Autodesk Inventor part; units mm, degrees
ref_plane "YZ Plane" through (0, 0, 0) normal (1, 0, 0) x (0, 1, 0)
ref_plane "XZ Plane" through (0, 0, 0) normal (0, 1, 0) x (-1, 0, 0)
ref_plane "XY Plane" through (0, 0, 0) normal (0, 0, 1) x (1, 0, 0)
sketch "Sketch1" plane through (0, 0, 0) normal (1, 0, 0) x (0, 1, 0)
  circle A0 centre (0, 0) radius 4.2
  circle A1 centre (0, 0) radius 6
  dimension "d0" = 8.4
  dimension "d1" = 12
extrude "Extrusion1" add sketch "Sketch1" along normal blind 8
sketch "Sketch2" plane through (8, 0, 0) normal (1, 0, 0) x (0, 0, -1)
  circle A0 centre (0, 0) radius 8.5
  circle A1 centre (0, 0) radius 4.2
  dimension "d4" = 17
extrude "Extrusion2" add sketch "Sketch2" along normal blind 5
fillet "Fillet1" radius 2 2 edges at (8, 0, 8.5) (8, -6, 0)
properties part number "Adaptador_Perno_Cojinete" material "ABS Plastic"
The listing builds one solid part. Answer for the finished solid, in the listing's coordinates (mm). A direction names the side the tool comes from. Round coordinates to 2 decimals unless told otherwise and drop trailing zeros. Order: outer loops, then holes, each group sorted by start corner. A loop starts at its lowest first (then second) coordinate and runs counter-clockwise, first axis right, second up. Notation, with made-up numbers: (73.25, 28) -> (88.25, 28) arc R29 cw to (88.25, 54) -> close; hole circle Ø6 at (-19, 62.5). An arc over 180 degrees is marked (long way). Put each result on its own line as item: value.
Q1. Determine the mould class of faces 3 (the flat face through (0, 3, -4)), 4 (the cylindrical face through (11.479, -7.167, -4.57)), 5 (the cylindrical face through (6.409, 1.981, -3.703)) for opening direction Z: pulls with the +Z half, pulls with the -Z half, needs draft (parallel to the pull), parting line crosses it, or undercut.
Results list:
face 3: needs draft
face 4: parting line crosses it
face 5: undercut
Q2. Which of the six approach directions +Z, -Z, +X, -X, +Y, -Y give full straight-line access (tool end or side, diameter ignored) to faces 1 (the flat face through (13, 4, -2)), 2 (the cylindrical face through (3, -6, 0))?
Results list:
face 1: +Z, -Z, +X, +Y, -Y
face 2: -X
Q3. Section A-A, the plane z = 0 is taken. Write down the section's boundary in (x, y).
Results list:
outline: (0, -6) -> (6.29, -6) arc R2 cw to (8.15, -7.25) arc R2 ccw to (10, -8.5) -> (13, -8.5) -> (13, -4.2) -> (0, -4.2) -> close; (0, 4.2) -> (13, 4.2) -> (13, 8.5) -> (10, 8.5) arc R2 ccw to (8.15, 7.25) arc R2 cw to (6.29, 6) -> (0, 6) -> close
Q4. Consider line 1 along Z through (x, y) = (4.75, 0); line 2 along Y through (x, z) = (10, 0); line 3 along Y through (x, z) = (5.75, 3.75). Determine where each line is inside the solid, lowest interval first.
Results list:
line 1: -6 to -4.2, 4.2 to 6
line 2: -8.5 to -4.2, 4.2 to 8.5
line 3: -4.68 to -1.89, 1.89 to 4.68
Q5. Section C-C, the plane x = 4 is taken. Write down the section's boundary in (y, z), and give its area (3 significant figures).
Results list:
outline: circle Ø12 at (0, 0); hole circle Ø8.4 at (0, 0)
area: 57.7 mm^2
Q6. Section D-D, the plane x = 9.5 is taken. Write down the section's boundary in (y, z), and give its area (3 significant figures).
Results list:
outline: circle Ø16.87 at (0, 0); hole circle Ø8.4 at (0, 0)
area: 168 mm^2
Q7. Each of these flat-tipped pins is pushed along its axis until it touches: P1, Ø4, axis at x = 7, y = -5.5, coming from the +Z side; P2, Ø4, axis at x = 2, z = 0.5, coming from the +Y side; P3, Ø1, axis at x = 5, y = -0.5, coming from the +Z side. Where does it stop, or does it pass through?
Results list:
P1: z = 6.67
P2: y = 6
P3: z = 6
